Work out the finished part from the listing and answer in its coordinate system (mm). Face numbers are marked on the shaded views. A direction names the side the tool comes from. Give positions to 0.01 mm unless a question says otherwise; leave off trailing zeros. Loops run counter-clockwise (first coordinate to the right, second up) from the corner with the lowest first, then second, coordinate; pieces in that order, holes last. Notation, with made-up numbers: M -28.75,43 L 19.25,43 A22 ccw 19.25,53 Z; hole C -29,14.25 d4. An arc over 180 degrees is marked long. Write item = value, one per line. Start each with the question number.
1. Section A-A on x = 47 is taken. Determine the outline of the cut face in (y, z).
2. Section C-C on y = 43 is taken. Determine the outline of the cut face in (x, z), plus the area to 3 significant figures.
3. Section D-D on x = -29 is taken. Determine the outline of the cut face in (y, z).
4. Section B-B on y = 9 is taken. Determine the outline of the cut face in (x, z).
5. For the marked faces 4 and 5, determine the directions among +Z, -Z, +X, -X, +Y, -Y from which every point of the face is accessible in a straight line to the end or side of a thin tool.
6. The mould has two halves that part along Z. Classify the marked faces 1, 2 and 3: released by +Z, released by -Z, zero draft, split by the parting line, or undercut.
7. Consider L1, parallel to Y at x = 95, z = -60; L2, parallel to X at y = 2, z = -42; L3, parallel to X at y = 3.35, z = 37.5. Determine where each line is inside the solid, lowest interval first. Write a range as [from, to].
8. Flat-ended cylindrical pins translate along their axes: pin 1 Ø2.5 at (x, z) = (-48.5, -61) entering from +Y; pin 2 Ø12 at (x, y) = (-5.5, 22) entering from -Z; pin 3 Ø1.5 at (y, z) = (48, 64.5) entering from -X; pin 4 Ø2.5 at (x, z) = (64, -42.5) entering from +Y. Find the tip coordinate at first contact, or state that the pin passes through.
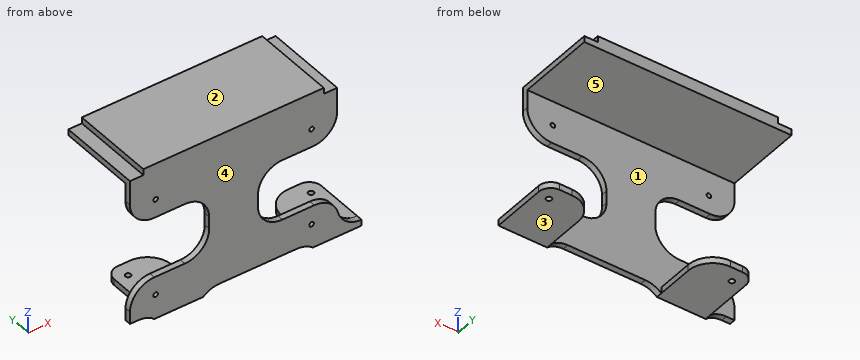
```python
from build123d import *

# Parameters (mm, degrees)
SKETCH1_R           = 1.9
BOSS_EXTRUDE1_DEPTH = 5
SKETCH1_4_W         = 148
SKETCH1_4_H         = 5
BOSS_EXTRUDE3_DEPTH = 69
SKETCH1_5_W         = 150
SKETCH1_5_H         = 5
SKETCH1_5_W_2       = 20
BOSS_EXTRUDE4_DEPTH = 55
SKETCH2_R           = 2.25
CUT_EXTRUDE1_DEPTH  = 60
FILLET1_R           = 20
FILLET2_R           = 10
SKETCH4_W           = 90
SKETCH4_H           = 5
CUT_EXTRUDE2_DEPTH  = 55
FILLET3_R           = 20


# Some blends are built 0.0001 mm under size
with BuildPart() as part:
    # Sketch1 → Boss-Extrude1 (new body)
    with BuildSketch(Plane(origin=(0, 0, 0), x_dir=(1, 0, 0), z_dir=(0, 1, 0))):
        Polygon((-85, -22.5), (-85, -57.5), (85, -57.5), (85, -22.5), (20, -22.5), (20, 27.5), (85, 27.5), (85, 57.5), (-65, 57.5), (-85, 57.5), (-85, 27.5), (-20, 27.5), (-20, -22.5), align=None)
        with Locations(Location((-64, -37.5, 0), (0, 0, 270))):
            Circle(SKETCH1_R, mode=Mode.SUBTRACT)
        with Locations(Location((64, -37.5, 0), (0, 0, 270))):
            Circle(SKETCH1_R, mode=Mode.SUBTRACT)
        with Locations(Location((-64, 42.5, 0), (0, 0, 270))):
            Circle(SKETCH1_R, mode=Mode.SUBTRACT)
        with Locations(Location((64, 42.5, 0), (0, 0, 270))):
            Circle(SKETCH1_R, mode=Mode.SUBTRACT)
    extrude(amount=BOSS_EXTRUDE1_DEPTH)

    # Sketch1<4> → Boss-Extrude3 (add)
    with BuildSketch(Plane(origin=(0, 0, 0), x_dir=(1, 0, 0), z_dir=(0, 1, 0))):
        with Locations((0, -65)):
            Rectangle(SKETCH1_4_W, SKETCH1_4_H)
        Polygon((85, -57.5), (-85, -57.5), (-85, -62.5), (-74, -62.5), (74, -62.5), (85, -62.5), align=None)
    extrude(amount=BOSS_EXTRUDE3_DEPTH)

    # Sketch1<5> → Boss-Extrude4 (add)
    with BuildSketch(Plane(origin=(0, 0, 0), x_dir=(1, 0, 0), z_dir=(0, 1, 0))):
        with Locations((10, 60)):
            Rectangle(SKETCH1_5_W, SKETCH1_5_H)
        with Locations((95, 60)):
            Rectangle(SKETCH1_5_W_2, SKETCH1_5_H)
    extrude(amount=BOSS_EXTRUDE4_DEPTH)

    # Sketch2 → Cut-Extrude1 (cut)
    with BuildSketch(Plane(origin=(0, 0, -62.5), x_dir=(-1, 0, 0), z_dir=(0, 0, -1))):
        with Locations((-95, 43)):
            Circle(SKETCH2_R)
        with Locations((55, 43)):
            Circle(SKETCH2_R)
    extrude(amount=-CUT_EXTRUDE1_DEPTH, mode=Mode.SUBTRACT)

    # Fillet1
    fillet1_edges = [part.edges().sort_by_distance(p)[0] for p in [
        (85, 2.5, -57.5),
    ]]
    fillet(fillet1_edges, radius=FILLET1_R - 0.0001)  # a hair under: the kernel refuses the full size

    # Fillet2
    fillet2_edges = [part.edges().sort_by_distance(p)[0] for p in [
        (-65, 55, -60),
        (105, 55, -60),
    ]]
    fillet(fillet2_edges, radius=FILLET2_R)

    # Sketch4 → Cut-Extrude2 (cut)
    with BuildSketch(Plane(origin=(0, 55, 0), x_dir=(1, 0, 0), z_dir=(0, 1, 0))):
        with Locations((20, 60)):
            Rectangle(SKETCH4_W, SKETCH4_H)
    extrude(amount=-CUT_EXTRUDE2_DEPTH, mode=Mode.SUBTRACT)

    # Fillet3
    # the kernel refuses this fillet: 20 mm, written as the material it adds along each edge
    with BuildSketch(Plane(origin=(65, 5, -57.5), x_dir=(-1, 0, 0), z_dir=(0, -1, 0))) as fillet3_piece_1:
        with BuildLine():
            CenterArc((13.228756555, 20), FILLET3_R, 228.590377891, 41.409622109)
            Line((0, 5), (0, 0))
            Line((0, 0), (13.228756555, 0))
        make_face()
    extrude(amount=5)
    with BuildSketch(Plane(origin=(-25, 5, -57.5), x_dir=(0, 0, -1), z_dir=(0, -1, 0)), Plane(origin=(-65, 0, -57.5), x_dir=(0, 0, -1), z_dir=(0, 1, 0))) as fillet3_piece_2:
        with BuildLine():
            CenterArc((20, 13.228756555), FILLET3_R, 180, 41.409622109)
            Line((0, 13.228756555), (0, 0))
            Line((0, 0), (5, 0))
        make_face()
    extrude(amount=5)
    with BuildSketch(Plane(origin=(-20, 0, 22.5), x_dir=(-1, 0, 0), z_dir=(0, 1, 0)), Plane(origin=(-20, 0, -27.5), x_dir=(0, 0, 1), z_dir=(0, 1, 0)), Plane(origin=(20, 0, 22.5), x_dir=(0, 0, -1), z_dir=(0, 1, 0)), Plane(origin=(20, 0, -27.5), x_dir=(1, 0, 0), z_dir=(0, 1, 0))) as fillet3_piece_3:
        with BuildLine():
            CenterArc((FILLET3_R, -FILLET3_R), FILLET3_R, 90, 90)
            Line((0, -FILLET3_R), (0, 0))
            Line((0, 0), (FILLET3_R, 0))
        make_face()
    extrude(amount=5)
    # the kernel refuses this fillet: 20 mm, written as the material it takes off along each edge
    with BuildSketch(Plane(origin=(-25, 55, -7.5), x_dir=(0, -1, 0), z_dir=(0, 0, -1)), Plane(origin=(65, 55, -112.5), x_dir=(0, -1, 0), z_dir=(0, 0, 1))) as fillet3_2_piece_1:
        with BuildLine():
            CenterArc((FILLET3_R, FILLET3_R), FILLET3_R, 180, 90)
            Line((0, FILLET3_R), (0, 0))
            Line((0, 0), (FILLET3_R, 0))
        make_face()
    extrude(amount=105, mode=Mode.SUBTRACT)
    with BuildSketch(Plane(origin=(85, -46.824640006, -27.5), x_dir=(0.04230002714791386, 0, -0.999104953297343), z_dir=(0, 1, 0))) as fillet3_2_piece_2:
        with BuildLine():
            CenterArc((19.189825649, 19.559092449), FILLET3_R, 182.42433637, 75.522598767)
            Line((-0.792273417, 18.713091906), (-2.790483324, 18.628491852))
            Line((-2.790483324, 18.628491852), (-1.998209907, -0.084600054))
            Line((-1.998209907, -0.084600054), (0.084600054, -1.998209907))
            ThreePointArc((0.084600054, -1.998209907), (10.075749498, -1.575205405), (14.595840223, -1.955909245))
            Line((14.595840223, -1.955909245), (15.013475262, 0))
        make_face()
    extrude(amount=98.649280012, mode=Mode.SUBTRACT)
    with BuildSketch(Plane(origin=(-85, -50, -27.5), x_dir=(0, 0, -1), z_dir=(0, 1, 0)), Plane(origin=(-85, -50, 22.5), x_dir=(1, 0, 0), z_dir=(0, 1, 0)), Plane(origin=(85, -50, 22.5), x_dir=(0, 0, 1), z_dir=(0, 1, 0))) as fillet3_2_piece_3:
        with BuildLine():
            CenterArc((FILLET3_R, -FILLET3_R), FILLET3_R, 90, 90)
            Line((0, -FILLET3_R), (0, 0))
            Line((0, 0), (FILLET3_R, 0))
        make_face()
    extrude(amount=105, mode=Mode.SUBTRACT)


solid = part.part
```
Verdict:
q1.outline = M 0,-57.5 L 5,-57.5 L 5,-27.5 L 0,-27.5 Z; M 0,22.5 L 5,22.5 L 5,57.5 L 69,57.5 L 69,67.5 L 0,67.5 Z
q2.outline = M -85,57.5 L 85,57.5 L 85,62.5 L 74,62.5 L 74,67.5 L -74,67.5 L -74,62.5 L -85,62.5 Z; M -65,-62.5 L -57.25,-62.5 L -57.25,-57.5 L -65,-57.5 Z; M -52.75,-62.5 L -26.67,-62.5 L -26.67,-57.5 L -52.75,-57.5 Z; M 66.67,-62.5 L 92.75,-62.5 L 92.75,-57.5 L 66.67,-57.5 Z; M 97.25,-62.5 L 105,-62.5 L 105,-57.5 L 97.25,-57.5 Z
q2.area = 1,930 mm2
q3.outline = M 0,-62.5 L 47,-62.5 L 47,-57.5 L 5,-57.5 L 5,-24.2 L 0,-24.2 Z; M 0,19.2 L 5,19.2 L 5,57.5 L 69,57.5 L 69,67.5 L 0,67.5 Z
q4.outline = M -85,57.5 L 85,57.5 L 85,62.5 L 74,62.5 L 74,67.5 L -74,67.5 L -74,62.5 L -85,62.5 Z; M -65,-62.5 L -25,-62.5 L -25,-57.5 L -65,-57.5 Z; M 65,-62.5 L 105,-62.5 L 105,-57.5 L 65,-57.5 Z
q5.face_4 = +Z, -Z, +X, -X, -Y
q5.face_5 = +X, -X, +Y
q6.face_1 = undercut
q6.face_2 = released by +Z
q6.face_3 = released by -Z
q7.L1 = [0, 40.75], [45.25, 55]
q7.L2 = [-84.23, -65.83], [-62.17, 62.17], [65.83, 85.5]
q7.L3 = [-84.36, -65.9], [-62.1, 62.1], [65.9, 84.36]
q8.pin_1 = 55
q8.pin_2 = 57.5
q8.pin_3 = -74
q8.pin_4 = through
